```python
from build123d import *

# Parameters (mm, degrees)
SKETCH_1_R          = 3
SKETCH_1_R_2        = 2
EXTRUDE_1_DEPTH     = 5
SKETCH_2_R          = 0.5
EXTRUDE_2_DEPTH     = 3.5
SKETCH_3_R          = 2
CUT_EXTRUDE_1_DEPTH = 3.5


with BuildPart() as part:
    # 草图1 → 凸台-拉伸1 (new body)
    with BuildSketch(Plane.XY):
        Circle(SKETCH_1_R)
        Circle(SKETCH_1_R_2, mode=Mode.SUBTRACT)
    extrude(amount=EXTRUDE_1_DEPTH)

    # 草图2 → 凸台-拉伸2 (add)
    with BuildSketch(Plane(origin=(0, 0, 0), x_dir=(1, 0, 0), z_dir=(0, 1, 0))):
        with Locations((0, -2.5)):
            Circle(SKETCH_2_R)
    extrude(amount=EXTRUDE_2_DEPTH)

    # 草图3 → 切除-拉伸1 (cut)
    with BuildSketch(Plane.XY.offset(5)):
        Circle(SKETCH_3_R)
    extrude(amount=-CUT_EXTRUDE_1_DEPTH, mode=Mode.SUBTRACT)


solid = part.part
```
Verification items for the finished model (mm, model axes). A direction names the side the tool comes from. Give positions to 0.01 mm unless a question says otherwise; leave off trailing zeros. Write each loop counter-clockwise with the first axis right and the second up, starting at its lowest first coordinate (ties: lowest second). Pieces come first, ordered by that corner, then holes. Notation, with made-up numbers: M 70,-26.5 L 76,-26.5 A25 cw 76,-6.5 Z; hole C 52.25,24.25 d2. An arc over 180 degrees is marked long. One line per question, with ' | ' between items.
1) Section check D-D on x = 1.75. Enter the section's corners in (y, z).
Result:
outline: M -2.44,0 L -0.97,0 L -0.97,5 L -2.44,5 Z; M 0.97,0 L 2.44,0 L 2.44,5 L 0.97,5 Z
2) Section check B-B on x = 0. Enter the section's corners in (y, z), plus the area to 3 significant figures.
Result:
outline: M -3,0 L -2,0 L -2,5 L -3,5 Z; M 2,0 L 3,0 L 3,2 L 3.5,2 L 3.5,3 L 3,3 L 3,5 L 2,5 Z | area: 10.5 mm2
3) Set-up check for faces 1 (the cylindrical face through (-0.5, 3.2, 2.5)), 2 (the flat face through (1, -2, 0)): record each of +Z, -Z, +X, -X, +Y, -Y from which the full face is reachable in a straight line by a thin tool's end or side.
Result:
face 1: +Y | face 2: -Z, +X, -X, +Y, -Y
4) Thickness scan on line 1 along Y through (x, z) = (0, 3.25); line 2 along Y through (x, z) = (0, 2.05); line 3 along X through (y, z) = (1.5, 3). Record the ranges inside material, lowest first. Write a range as [from, to].
Result:
line 1: y = [-3, -2], [2, 3] | line 2: y = [-3, -2], [2, 3.5] | line 3: x = [-2.6, -1.32], [1.32, 2.6]
5) Section check C-C on z = 2.5. Enter the section's corners in (x, y), plus the area to 3 significant figures.
Result:
outline: M -0.5,2.96 A3 ccw long 0.5,2.96 L 0.5,3.5 L -0.5,3.5 Z; hole C 0,0 d4 | area: 16.2 mm2
6) Section check A-A on y = 0. Enter the section's corners in (x, z), plus the area to 3 significant figures.
Result:
outline: M -3,0 L -2,0 L -2,5 L -3,5 Z; M 2,0 L 3,0 L 3,5 L 2,5 Z | area: 10.0 mm2
